```python
from build123d import *

# Parameters (mm, degrees)
SKETCH4_R           = 75
BOSS_EXTRUDE2_DEPTH = 15
CUT_EXTRUDE1_DEPTH  = 108.121426428
CIRPATTERN1_COUNT   = 4
SHELL1_DEPTH        = 13
SKETCH7_R           = 12.503328754
BOSS_EXTRUDE3_DEPTH = 12.5
SKETCH8_R           = 3.25
SKETCH8_R_2         = 2.25
BOSS_EXTRUDE4_DEPTH = 8.5
CUT_EXTRUDE2_START  = -10
SKETCH9_R           = 12.503328754
SKETCH9_R_2         = 3.25
CUT_EXTRUDE2_DEPTH  = 10


# Read off the part's stored shape, not the designer's step: Shell1
with BuildPart() as part:
    # Sketch4 → Boss-Extrude2 (new body)
    with BuildSketch(Plane.XY):
        Circle(SKETCH4_R)
    extrude(amount=BOSS_EXTRUDE2_DEPTH)

    # Sketch6 → Cut-Extrude1 (cut, symmetric)
    with BuildSketch(Plane.XY):
        with BuildLine():
            Line((2.206615595, 15), (2.206615595, 69.72932719))
            Line((2.206615595, 69.72932719), (2.206615595, 72.96664202))
            ThreePointArc((2.206615595, 72.96664202), (51.691823279, 51.54566331), (72.972597597, 2))
            Line((72.972597597, 2), (15, 2))
            Line((15, 2), (14.866068747, 2))
            ThreePointArc((14.866068747, 2), (10.680123706, 10.532566526), (2.206615595, 14.836807191))
            Line((2.206615595, 14.836807191), (2.206615595, 15))
        make_face()
    cut_extrude1 = extrude(amount=CUT_EXTRUDE1_DEPTH, both=True, mode=Mode.SUBTRACT)

    # CirPattern1: Cut-Extrude1 ×4 about axis
    cirpattern1_axis = Axis((0, 0, 0), (0, 0, 1))
    for i in range(1, CIRPATTERN1_COUNT):
        add(cut_extrude1.rotate(cirpattern1_axis, i * 360 / CIRPATTERN1_COUNT), mode=Mode.SUBTRACT)

    # Shell1 outline → Shell1 (cut)
    with BuildSketch(Plane.XY):
        with BuildLine():
            ThreePointArc((-0.206615595, -72.999707602), (-0.103307901, -72.9999269), (0, -73))
            Line((0, -73), (0, -13))
            ThreePointArc((0, -13), (9.119045928, -9.26514983), (12.998357973, -0.206615595))
            Line((12.998357973, -0.206615595), (72.999707602, -0.206615595))
            ThreePointArc((72.999707602, -0.206615595), (72.9999269, -0.103307901), (73, 0))
            Line((73, 0), (13, 0))
            ThreePointArc((13, 0), (9.26514983, 9.119045928), (0.206615595, 12.998357973))
            Line((0.206615595, 12.998357973), (0.206615595, 72.999707602))
            ThreePointArc((0.206615595, 72.999707602), (0.103307901, 72.9999269), (0, 73))
            Line((0, 73), (0, 13))
            ThreePointArc((0, 13), (-9.119045928, 9.26514983), (-12.998357973, 0.206615595))
            Line((-12.998357973, 0.206615595), (-72.999707602, 0.206615595))
            ThreePointArc((-72.999707602, 0.206615595), (-72.9999269, 0.103307901), (-73, 0))
            Line((-73, 0), (-13, 0))
            ThreePointArc((-13, 0), (-9.26514983, -9.119045928), (-0.206615595, -12.998357973))
            Line((-0.206615595, -12.998357973), (-0.206615595, -72.999707602))
        make_face()
    extrude(amount=SHELL1_DEPTH, mode=Mode.SUBTRACT)

    # Sketch7 → Boss-Extrude3 (add)
    with BuildSketch(Plane(origin=(0, 0, 13), x_dir=(-1, 0, 0), z_dir=(0, 0, -1))):
        with Locations(Location((0, 0, 0), (0, 0, 180))):
            Circle(SKETCH7_R)
    extrude(amount=BOSS_EXTRUDE3_DEPTH)

    # Sketch8 → Boss-Extrude4 (add)
    with BuildSketch(Plane(origin=(0, 0, 0.5), x_dir=(-1, 0, 0), z_dir=(0, 0, -1))):
        Circle(SKETCH8_R)
        Circle(SKETCH8_R_2, mode=Mode.SUBTRACT)
    extrude(amount=BOSS_EXTRUDE4_DEPTH)

    # Sketch9 → Cut-Extrude2 (cut)
    with BuildSketch(Plane(origin=(0, 0, 0.5), x_dir=(-1, 0, 0), z_dir=(0, 0, -1)).offset(CUT_EXTRUDE2_START)):
        with Locations(Location((0, 0, 0), (0, 0, 180))):
            Circle(SKETCH9_R)
        Circle(SKETCH9_R_2, mode=Mode.SUBTRACT)
    extrude(amount=CUT_EXTRUDE2_DEPTH, mode=Mode.SUBTRACT)


solid = part.part
```
Input: part model. Units: mm. Frame: model coordinates. A direction names the side the tool comes from. Round coordinates to 2 decimals unless told otherwise and drop trailing zeros. Write each loop counter-clockwise with the first axis right and the second up, starting at its lowest first coordinate (ties: lowest second). Pieces come first, ordered by that corner, then holes. Notation, with made-up numbers: (48.5, 14) -> (93.5, 14) arc R32 cw to (93.5, 51) -> close; hole circle Ø6 at (34.5, -19). An arc over 180 degrees is marked (long way). Answer as CSV lines item,"result".
1. Mould query, pull axis X, two halves, no side actions, for faces 3 (the cylindrical face through (-9.764, 74.362, 7.395)), 4 (the flat face through (-43, 0, 6)), 5 (the flat face through (0, 0, 15)), 6 (the flat face through (-2, 44, 8)). Classes: +X half, -X half, draft (parallel to the pull), parting line (faces both ways), or undercut.
Geometry says:
face 3,"parting line"
face 4,"undercut"
face 5,"draft"
face 6,"undercut"
2. Section A-A (z = 3.75). Give the number of separate pieces and of enclosed holes in the cut face, plus the area to 3 significant figures.
Geometry says:
separate pieces,"2"
enclosed holes,"5"
area,"2,070 mm^2"
3. Reachability of faces 1 (the cylindrical face through (52.09, -51.143, 7.605)), 2 (the cylindrical face through (9.02, -9.36, 6.41)) from +Z, -Z, +X, -X, +Y, -Y: full face, straight path, thin tool, end or side. Return the list, or none.
Geometry says:
face 1,"+Z, -Z"
face 2,"-Z"
4. Ray query, L1, parallel to Y at x = 0, z = -4; L2, parallel to Y at x = 1.5, z = 1.5 (3 decimals); L3, parallel to Y at x = 47, z = 1.25. Return the intervals inside material, ascending. Write a range as [from, to].
Geometry says:
L1,"y = [-3.25, -2.25], [2.25, 3.25]"
L2,"y = [-74.985, -12.913], [-2.883, 2.883], [12.913, 74.985]"
L3,"y = [-58.45, -55.86], [-2.21, -0.21], [0, 2], [55.86, 58.45]"
5. Contact query for flat-ended pins moving along their axis: P1, Ø2, axis at x = 4, z = 9, coming from the -Y side; P2, Ø6, axis at x = -0.5, z = 8, coming from the +Y side; P3, Ø10.5, axis at x = 55.5, z = 9, coming from the +Y side. Output: stop coordinate, or through.
Geometry says:
P1,"stops at y = -74.94"
P2,"stops at y = 75"
P3,"stops at y = 55.68"
6. Section B-B (y = -18). Return the cut outline in (x, z).
Geometry says:
outline,"(-72.81, 0) -> (-70.75, 0) -> (-70.75, 15) -> (-72.81, 15) -> close; (-2.21, 0) -> (-0.21, 0) -> (-0.21, 13) -> (0, 13) -> (0, 0) -> (2, 0) -> (2, 15) -> (-2.21, 15) -> close; (70.75, 0) -> (72.81, 0) -> (72.81, 15) -> (70.75, 15) -> close"
7. Section C-C (y = -63). Return the cut outline in (x, z), plus the area to 3 significant figures.
Geometry says:
outline,"(-40.69, 0) -> (-36.88, 0) -> (-36.88, 15) -> (-40.69, 15) -> close; (-2.21, 0) -> (-0.21, 0) -> (-0.21, 13) -> (0, 13) -> (0, 0) -> (2, 0) -> (2, 15) -> (-2.21, 15) -> close; (36.88, 0) -> (40.69, 0) -> (40.69, 15) -> (36.88, 15) -> close"
area,"175 mm^2"
